Could you check a few things on this model? Use its own coordinates, in mm. A direction names the side the tool comes from. Round coordinates to 2 decimals unless told otherwise and drop trailing zeros. Write each loop counter-clockwise with the first axis right and the second up, starting at its lowest first coordinate (ties: lowest second). Pieces come first, ordered by that corner, then holes. Notation, with made-up numbers: (29.25, 43) -> (72.25, 43) arc R13 ccw to (72.25, 66) -> close; hole circle Ø7 at (-4, 65.25). An arc over 180 degrees is marked (long way). One line per question, with ' | ' between items. Start each with the question number.
1. Imagine slicing it at A-A, the plane x = 0. List the corners of the cut face in (y, z) for me.
2. Imagine slicing it at C-C, the plane y = -2. List the corners of the cut face in (x, z) for me.
3. Imagine slicing it at B-B, the plane z = 0.4. State how many separate pieces and enclosed holes the cut face has, and give its area (3 significant figures).
4. For pin 1 Ø4.5 at (x, y) = (0, -8.5) entering from +Z, with a flat end and sliding along its axis, tell me the tip position at first contact or that it passes through.
5. Imagine slicing it at D-D, the plane x = -8.5. List the corners of the cut face in (y, z) for me, and give its area (3 significant figures).
6. If I drill on line 1 along Y through (x, z) = (-30, 1.55); line 2 along Y through (x, z) = (0, 0.6); line 3 along Y through (x, z) = (-26.5, 1.7), over which ranges is the centre line in solid material (lowest first)? Write a range as [from, to].
7. For faces 4 (the cylindrical face through (11.5, 0.2, 1)), 5 (the flat face through (-29, -6.05, 1)), which set-ups out of +Z, -Z, +X, -X, +Y, -Y let a thin tool reach every point of the face, with its end or its side?
8. Thinking about a two-plate mould opening in Y: for faces 1 (the flat face through (-30, 16, 1)), 2 (the flat face through (-16, 0, 0)), 3 (the flat face through (-30.05, 0, 1)), which applies, released by +Y, released by -Y, zero draft, split by the parting line, or undercut?
Autodesk Inventor part; units mm, degrees
ref_plane "YZ Plane" through (0, 0, 0) normal (1, 0, 0) x (0, 1, 0)
ref_plane "XZ Plane" through (0, 0, 0) normal (0, 1, 0) x (-1, 0, 0)
ref_plane "XY Plane" through (0, 0, 0) normal (0, 0, 1) x (1, 0, 0)
sketch "スケッチ1" plane through (0, 0, 0) normal (0, 0, 1) x (1, 0, 0)
  circle A0 centre (0, 0) radius 10.5 construction
  circle A1 centre (0, 8.5) radius 1.35
  circle A2 centre (-8.5, 0) radius 1.35
  circle A3 centre (0, -8.5) radius 1.35
  circle A4 centre (8.5, 0) radius 1.35
  circle A5 centre (0, 0) radius 5.05
  line L0 (-30, 6) -> (-27.5, 6) construction
  line L1 (-27.5, 6) -> (-27.5, -6) construction
  line L2 (-27.5, -6) -> (-30, -6) construction
  line L3 (-30, -6) -> (-30, 6) construction
  line L4 (-27.45, 6.05) -> (-30.05, 6.05) construction
  line L5 (-30.05, 6.05) -> (-30.05, -6.05) construction
  line L6 (-30.05, -6.05) -> (-27.45, -6.05) construction
  line L7 (-27.45, -6.05) -> (-27.45, 6.05) construction
  circle A6 centre (-30.05, 5) radius 1.05 construction
  line L8 (-27.45, 6.05) -> (-30.05, 6.05)
  arc A7 (-30.05, 6.05) -> (-30.05, 3.95) centre (-30.05, 5) ccw
  line L9 (-30.05, 3.95) -> (-30.05, -3.95)
  line L10 (-28.75, 6.05) -> (-28.75, -6.05) construction
  line L11 (-30.05, 0) -> (-27.5, 0) construction
  arc A8 (-30.05, -3.95) -> (-30.05, -6.05) centre (-30.05, -5) ccw
  line L12 (-30.05, -6.05) -> (-27.45, -6.05)
  line L13 (-27.45, 3.95) -> (-27.45, -3.95)
  arc A9 (-27.45, 3.95) -> (-27.45, 6.05) centre (-27.45, 5) ccw
  arc A10 (-27.45, -6.05) -> (-27.45, -3.95) centre (-27.45, -5) ccw
  circle A11 centre (-30, 12) radius 1.55
  circle A12 centre (-30, -12) radius 1.55
  line L14 (-32.5, 16) -> (-27.5, 16)
  line L15 (-32.5, -16) -> (-27.5, -16)
  arc A13 (1.7994, -11.3584) -> (1.7994, 11.3584) centre (0, 0) ccw
  line L16 (-32.5, 16) -> (-32.5, -16)
  line L17 (-27.5, 16) -> (1.7994, 11.3584)
  line L18 (1.7994, -11.3584) -> (-27.5, -16)
  point P0 (-28.775, 0)
  dimension "d29" = 2.1
  dimension "d0" = 21
  dimension "d3" = 8.5
  dimension "d4" = 2.7
  dimension "d7" = 360
  dimension "d9" = 10.1
  dimension "d10" = 2.5
  dimension "d30" = 0.05
  dimension "d31" = 6
  dimension "d33" = 3.1
  dimension "d43" = 1
  dimension "d57" = 32
  dimension "d61" = 32.5
  dimension "d62" = 5
  dimension "d63" = 2.5
  dimension "d65" = 10
extrude "押し出し1" add sketch "スケッチ1" along normal blind 2
equation "\"d23\" = 7"
properties part number "Shoulder_vertical_frame_02" material "アルミニウム 2014-T4"
Geometry results:
1) outline: (-11.64, 0) -> (-9.85, 0) -> (-9.85, 2) -> (-11.64, 2) -> close; (-7.15, 0) -> (-5.05, 0) -> (-5.05, 2) -> (-7.15, 2) -> close; (5.05, 0) -> (7.15, 0) -> (7.15, 2) -> (5.05, 2) -> close; (9.85, 0) -> (11.64, 0) -> (11.64, 2) -> (9.85, 2) -> close
2) outline: (-32.5, 0) -> (-30.05, 0) -> (-30.05, 2) -> (-32.5, 2) -> close; (-27.45, 0) -> (-4.64, 0) -> (-4.64, 2) -> (-27.45, 2) -> close; (4.64, 0) -> (11.32, 0) -> (11.32, 2) -> (4.64, 2) -> close
3) separate pieces: 1 | enclosed holes: 8 | area: 972 mm2
4) pin 1: stops at z = 2
5) outline: (-12.99, 0) -> (-1.35, 0) -> (-1.35, 2) -> (-12.99, 2) -> close; (1.35, 0) -> (12.99, 0) -> (12.99, 2) -> (1.35, 2) -> close | area: 46.6 mm2
6) line 1: y = [-16, -13.55], [-10.45, -6.05], [6.05, 10.45], [13.55, 16] | line 2: y = [-11.64, -9.85], [-7.15, -5.05], [5.05, 7.15], [9.85, 11.64] | line 3: y = [-15.84, -5.45], [-4.55, 4.55], [5.45, 15.84]
7) face 4: +Z, -Z, +X | face 5: +Z, -Z
8) face 1: released by +Y | face 2: zero draft | face 3: undercut
